Job drawing, mm, ordinate dimensions from the low corner. One solid piece. A direction names the side the tool comes from. Round coordinates to 2 decimals unless told otherwise and drop trailing zeros. Loops run counter-clockwise (first coordinate to the right, second up) from the corner with the lowest first, then second, coordinate; pieces in that order, holes last. Notation, with made-up numbers: (16, 29) - (25, 29) arc R28 ccw to (25, 47) - close; hole circle Ø6 at (0, -22.75). An arc over 180 degrees is marked (long way). Answer as CSV lines item,"result". Start each with the question number.
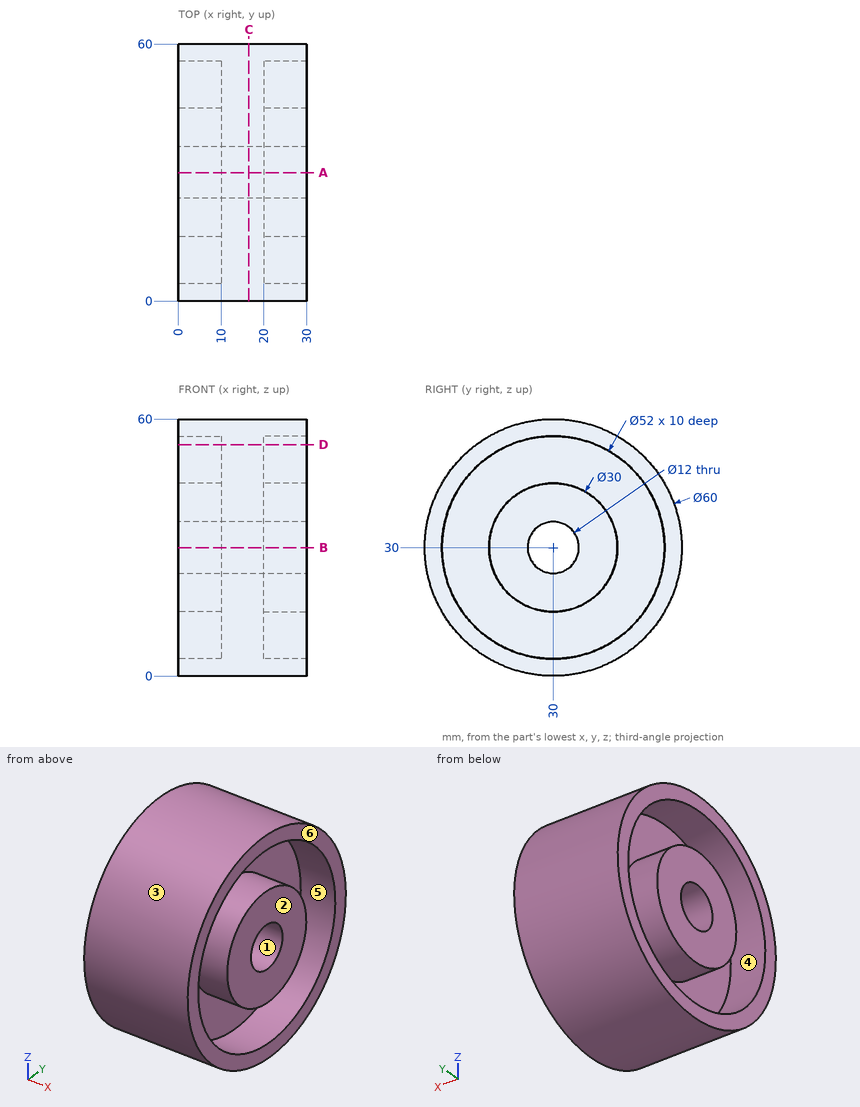
Q1. Band-saw the part on D-D, the plane z = 54. List the corners of the cut face in (x, y).
Q2. Band-saw the part on C-C, the plane x = 16.5. List the corners of the cut face in (y, z).
Q3. Tool access for the marked faces 4, 5 and 6: list every direction of +Z, -Z, +X, -X, +Y, -Y with a clear straight run to the whole face (end or side of a thin tool).
Q4. Band-saw the part on A-A, the plane y = 30. List the corners of the cut face in (x, z), then the cut area to 3 significant figures.
Q5. Two-plate mould, pull along Y, no slides. Class the marked faces 1, 2 and 3: released by +Y, released by -Y, zero draft, split by the parting line, or undercut.
Q6. Wall check: probe 1 along Y at (x, z) = (25, 30); probe 2 along Y at (x, z) = (2.5, 36.5); probe 3 along Y at (x, z) = (4.75, 18.5). Give the ranges that are in metal, low to high. Write a range as [from, to].
Q7. Pin check, flat tips, straight feed: pin 1 Ø1.5 at (x, y) = (12.5, 46) entering from -Z; pin 2 Ø5 at (y, z) = (15, 32) entering from -X; pin 3 Ø5 at (x, z) = (23, 22.5) entering from -Y; pin 4 Ø6 at (y, z) = (18, 12) entering from +X. Stop position of each tip, or through.
Reported:
1,outline,"(0, 12) - (30, 12) - (30, 20) - (20, 20) - (20, 40) - (30, 40) - (30, 48) - (0, 48) - (0, 40) - (10, 40) - (10, 20) - (0, 20) - close"
2,outline,"circle Ø60 at (30, 30); hole circle Ø12 at (30, 30)"
3,face 4,"-X"
3,face 5,"+X"
3,face 6,"+Z, -Z, +X, +Y, -Y"
4,outline,"(0, 0) - (30, 0) - (30, 4) - (20, 4) - (20, 15) - (30, 15) - (30, 24) - (0, 24) - (0, 15) - (10, 15) - (10, 4) - (0, 4) - close; (0, 36) - (30, 36) - (30, 45) - (20, 45) - (20, 56) - (30, 56) - (30, 60) - (0, 60) - (0, 56) - (10, 56) - (10, 45) - (0, 45) - close"
4,area,"1,000 mm2"
5,face 1,"undercut"
5,face 2,"zero draft"
5,face 3,"split by the parting line"
6,probe 1,"y = [0, 4], [15, 24], [36, 45], [56, 60]"
6,probe 2,"y = [0.71, 4.83], [16.48, 43.52], [55.17, 59.29]"
6,probe 3,"y = [2.29, 6.68], [20.37, 39.63], [53.32, 57.71]"
7,pin 1,"stops at z = 4.17"
7,pin 2,"stops at x = 0"
7,pin 3,"stops at y = 0.42"
7,pin 4,"stops at x = 20"
